Check sheet for the drawn part. Datum: minimum x, y, z corner. Units: mm. Coordinates: 2 decimals unless noted, no trailing zeros. Order: outer loops, then holes, each group sorted by start corner. A loop starts at its lowest first (then second) coordinate and runs counter-clockwise, first axis right, second up.
1. Cross-section at A-A (z = 2.75). Enter the section's corners in (x, y) (3 decimals).
2. Draft check along X on the marked faces 1 and 2. Enter one of: released by +X, released by -X, zero draft, split by the parting line, or undercut.
3. Cross-section at C-C (x = 38.1). Enter the section's corners in (y, z) (3 decimals), then the cut area to 3 significant figures.
4. Cross-section at D-D (x = 50.8). Enter the section's corners in (y, z) (3 decimals), then the cut area to 3 significant figures.
5. Thickness scan on line 1 (Z direction, x = 73, y = 16.5) (3 decimals); line 2 (X direction, y = 13, z = 4.25); line 3 (Y direction, x = 38, z = 11.25). Record the ranges inside material, lowest first.
6. Cross-section at B-B (y = 12.7). Enter the section's corners in (x, z) (3 decimals).
7. Gauge pin test, flat ends, axial feed: pin 1 Ø6 at (x, z) = (69, 9) entering from +Y; pin 2 Ø2 at (x, z) = (36, 18) entering from +Y; pin 3 Ø4 at (x, z) = (45, 17.5) entering from +Y; pin 4 Ø12 at (x, z) = (90, 10.5) entering from +Y. Record the tip position at first contact, or that the pin passes through.
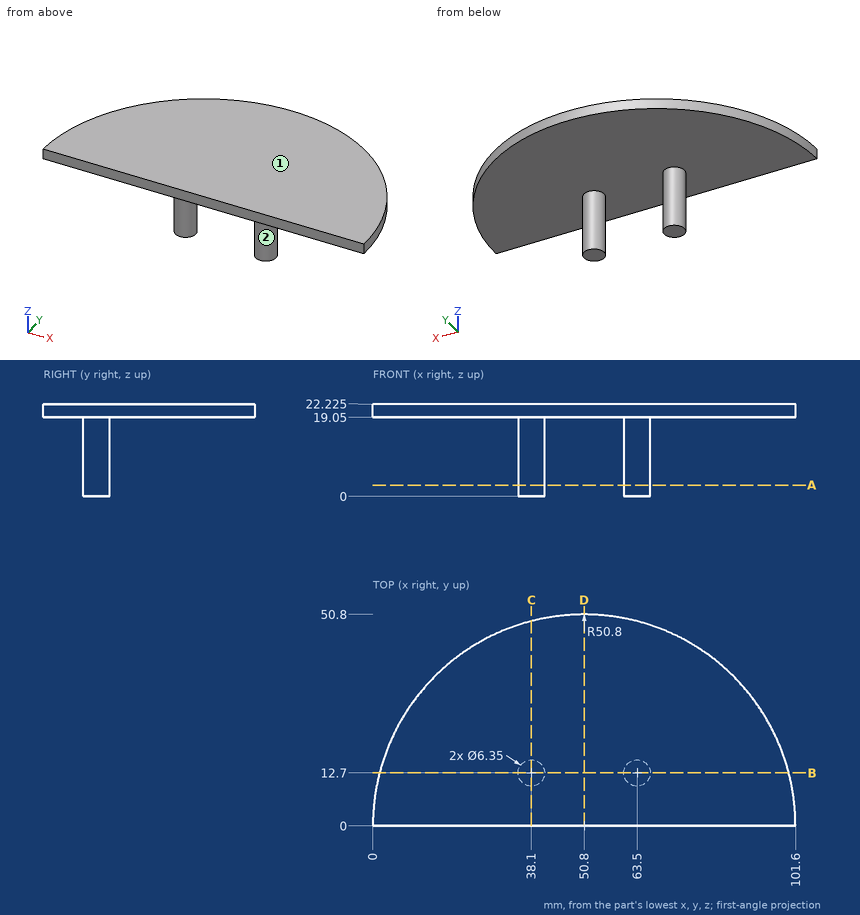
Data:
1. outline: circle Ø6.35 at (38.1, 12.7); circle Ø6.35 at (63.5, 12.7)
2. face 1: zero draft
2. face 2: undercut
3. outline: (0, 19.05) - (9.525, 19.05) - (9.525, 0) - (15.875, 0) - (15.875, 19.05) - (49.187, 19.05) - (49.187, 22.225) - (0, 22.225) - close
3. area: 277 mm2
4. outline: (0, 19.05) - (50.8, 19.05) - (50.8, 22.225) - (0, 22.225) - close
4. area: 161 mm2
5. line 1: z = 19.05 to 22.225
5. line 2: x = 34.94 to 41.26, 60.34 to 66.66
5. line 3: y = 9.53 to 15.87
6. outline: (1.613, 19.05) - (34.925, 19.05) - (34.925, 0) - (41.275, 0) - (41.275, 19.05) - (60.325, 19.05) - (60.325, 0) - (66.675, 0) - (66.675, 19.05) - (99.987, 19.05) - (99.987, 22.225) - (1.613, 22.225) - close
7. pin 1: stops at y = 14.66
7. pin 2: stops at y = 15.68
7. pin 3: stops at y = 50.6
7. pin 4: passes through
